Design review of the part built by this model. Coordinates are the model's own, in mm. A direction names the side the tool comes from. Coordinates: 2 decimals unless noted, no trailing zeros. Write item = value, one per line. Start each with the question number.
```python
from build123d import *

# Parameters (mm, degrees)
BASPROSKE_W             = 10
BASPROSKE_H             = 19
TOOTHCUT_DEPTH          = 29.670542374
TEETHCUTS_COUNT         = 17
TEETHCUTS_ANGLE         = 338.823529412
BORSKE_R                = 2.5
BORE_DEPTH              = 50.0008636
SKETCH1_W               = 10
SKETCH1_H               = 40
CUT_EXTRUDE1_DEPTH      = 20
CUT_EXTRUDE1_DEPTH_BACK = 20
CUT_EXTRUDE3_DEPTH      = 2.5
SKETCH3_R               = 1
CUT_EXTRUDE4_DEPTH      = 27.95667967


with BuildPart() as part:
    # BasProSke → Base-Revolve (revolve)
    with BuildSketch(Plane(origin=(0, 0, 0), x_dir=(1, 0, 0), z_dir=(0, 1, 0)), mode=Mode.PRIVATE) as base_revolve_sk:
        with Locations((5, 9.5)):
            Rectangle(BASPROSKE_W, BASPROSKE_H)
    revolve(base_revolve_sk.sketch.rotate(Axis((-10, 0, 0), (1, 0, 0)), 180), axis=Axis((-10, 0, 0), (1, 0, 0)))

    # TooCutSke → ToothCut (cut, through all)
    with BuildSketch(Plane(origin=(0, 0, 0), x_dir=(0, 0, -1), z_dir=(1, 0, 0))):
        with BuildLine():
            ThreePointArc((1.020352389, 14.463052306), (0, 14.499), (-1.020352389, 14.463052306))
            ThreePointArc((-1.020352389, 14.463052306), (-1.632621885, 16.804485203), (-3.026143023, 18.783192049))
            ThreePointArc((-3.026143023, 18.783192049), (0, 19.0254), (3.026143023, 18.783192049))
            ThreePointArc((3.026143023, 18.783192049), (1.632621885, 16.804485203), (1.020352389, 14.463052306))
        make_face()
    toothcut = extrude(amount=TOOTHCUT_DEPTH, mode=Mode.SUBTRACT)

    # TeethCuts: ToothCut ×17 about axis
    teethcuts_axis = Axis((-10, 0, 0), (1, 0, 0))
    for i in range(1, TEETHCUTS_COUNT):
        add(toothcut.rotate(teethcuts_axis, i * TEETHCUTS_ANGLE / (TEETHCUTS_COUNT - 1)), mode=Mode.SUBTRACT)

    # BorSke → Bore (cut, symmetric)
    with BuildSketch(Plane(origin=(0, 0, 0), x_dir=(0, 0, -1), z_dir=(1, 0, 0))):
        with Locations(Location((0, 0, 0), (0, 0, 180))):
            Circle(BORSKE_R)
    extrude(amount=BORE_DEPTH, both=True, mode=Mode.SUBTRACT)

    # Sketch1 → Cut-Extrude1 (cut, two sides)
    with BuildSketch(Plane.XY) as cut_extrude1_sk:
        Rectangle(SKETCH1_W, SKETCH1_H)
    extrude(amount=CUT_EXTRUDE1_DEPTH, mode=Mode.SUBTRACT)
    extrude(cut_extrude1_sk.sketch, amount=-CUT_EXTRUDE1_DEPTH_BACK, mode=Mode.SUBTRACT)

    # Sketch2 → Cut-Extrude3 (cut)
    with BuildSketch(Plane.ZY.offset(-5)):
        with BuildLine():
            Line((0, -16.5), (0, -12.5))
            ThreePointArc((0, -12.5), (-1.414213562, -13.085786438), (-2, -14.5))
            ThreePointArc((-2, -14.5), (-1.414213562, -15.914213562), (0, -16.5))
        make_face()
        with BuildLine():
            ThreePointArc((2, -14.5), (1.414213562, -13.085786438), (0, -12.5))
            Line((0, -12.5), (0, -16.5))
            ThreePointArc((0, -16.5), (1.414213562, -15.914213562), (2, -14.5))
        make_face()
        with BuildLine():
            ThreePointArc((3.850641774, -1.082847141), (2.415430752, -3.188368593), (0, -4))
            Line((0, -4), (0, -12.5))
            ThreePointArc((0, -12.5), (1.414213562, -13.085786438), (2, -14.5))
            Line((2, -14.5), (3.850641774, -1.082847141))
        make_face()
        with BuildLine():
            Line((0, -12.5), (0, -4))
            ThreePointArc((0, -4), (-2.624080254, -3.018973803), (-3.961014771, -0.557101411))
            Line((-3.961014771, -0.557101411), (-2, -14.5))
            ThreePointArc((-2, -14.5), (-1.414213562, -13.085786438), (0, -12.5))
        make_face()
        with BuildLine():
            ThreePointArc((-3.961014771, -0.557101411), (-2.624080254, -3.018973803), (0, -4))
            ThreePointArc((0, -4), (2.415430752, -3.188368593), (3.850641774, -1.082847141))
            Line((3.850641774, -1.082847141), (4, 0))
            ThreePointArc((4, 0), (-0.279231906, 3.99024179), (-3.961014771, -0.557101411))
        make_face()
        with BuildLine():
            ThreePointArc((2.5, 0), (1.767766953, -1.767766953), (0, -2.5))
            ThreePointArc((0, -2.5), (-1.767766953, 1.767766953), (2.5, 0))
        make_face(mode=Mode.SUBTRACT)
    extrude(amount=-CUT_EXTRUDE3_DEPTH, mode=Mode.SUBTRACT)

    # Sketch3 → Cut-Extrude4 (cut, through all)
    with BuildSketch(Plane.ZY.offset(-7.5)):
        with Locations(Location((0, -12.45, 0), (0, 0, 270))):
            Circle(SKETCH3_R)
        with Locations(Location((0, -8.45, 0), (0, 0, 270))):
            Circle(SKETCH3_R)
    extrude(amount=-CUT_EXTRUDE4_DEPTH, mode=Mode.SUBTRACT)


solid = part.part
```
Item 1: Mouldability with a two-part tool opening along Z and no side actions: class faces 4 (the cylindrical face through (7.54, 16.15, -10.01)), 5 (the cylindrical face through (7.465, 1.352, 14.436)), 6 (the flat face through (6.2, -7.4, -3)) as +Z half, -Z half, draft (parallel to the pull), parting line (faces both ways), or undercut.
Item 2: For faces 1 (the cylindrical face through (6, 4, 0)), 2 (the cylindrical face through (7.46, -15.16, -7.46)), 3 (the cylindrical face through (7.46, 15.05, 7.56)), list the 3-axis set-ups (+Z, -Z, +X, -X, +Y, -Y) from which the entire face can be reached by the end or side of a thin tool; tool diameter is ignored.
Item 3: For line 1 (Z direction, x = 8.2, y = -8.45); line 2 (Y direction, x = 7.2, z = 15.5); line 3 (Z direction, x = 7.2, y = 16), list the stretches that pass through material, from the lowest coordinate up.
Item 4: Add section A-A on x = 8.1. State how many separate pieces and enclosed holes the cut face has, plus the area to 3 significant figures.
Item 5: For P1, Ø2.5, axis at y = -8.45, z = 0, coming from the -X side; P2, Ø1.5, axis at x = 6.5, y = 8.5, coming from the -Z side; P3, Ø2, axis at x = 6.5, z = 6, coming from the +Y side, all flat-tipped, find the tip position at first contact; note any pin that passes through.
Worked out:
q1.face_4 = -Z half
q1.face_5 = +Z half
q1.face_6 = undercut
q2.face_1 = -X
q2.face_2 = +X, -X
q2.face_3 = +X, -X, +Y
q3.line_1 = -17.02 to -13.2, -11.78 to -1, 1 to 11.78, 13.2 to 17.02
q3.line_2 = -8.97 to -5.99, -3.11 to 0.26, 2.67 to 6.02
q3.line_3 = -10.25 to -8.79, -4.56 to -1.32, 1.32 to 4.56, 8.79 to 10.25
q4.separate_pieces = 1
q4.enclosed_holes = 3
q4.area = 845 mm2
q5.P1 = 7.5
q5.P2 = -14.54
q5.P3 = 14.43
